from build123d import *

# Parameters (mm, degrees)
SKETCH1_R           = 100
SKETCH1_R_2         = 45
BOSS_EXTRUDE1_DEPTH = 60
SKETCH2_R           = 45
BOSS_EXTRUDE2_DEPTH = 15
CUT_EXTRUDE2_DEPTH  = 85
SKETCH5_R           = 70
CUT_EXTRUDE3_DEPTH  = 5
CUT_EXTRUDE4_DEPTH  = 50


with BuildPart() as part:
    # Sketch1 → Boss-Extrude1 (new body)
    with BuildSketch(Plane(origin=(0, 0, 0), x_dir=(1, 0, 0), z_dir=(0, 1, 0))):
        with Locations(Location((0, 0, 0), (0, 0, 270))):
            Circle(SKETCH1_R)
        with Locations(Location((0, 0, 0), (0, 0, 270))):
            Circle(SKETCH1_R_2, mode=Mode.SUBTRACT)
    extrude(amount=BOSS_EXTRUDE1_DEPTH)

    # Sketch2 → Boss-Extrude2 (add)
    with BuildSketch(Plane.XZ):
        with Locations(Location((0, 0, 0), (0, 0, 270))):
            Circle(SKETCH2_R)
    extrude(amount=-BOSS_EXTRUDE2_DEPTH)

    # Sketch4 → Cut-Extrude2 (cut)
    with BuildSketch(Plane(origin=(0, 60, 0), x_dir=(1, 0, 0), z_dir=(0, 1, 0))):
        with BuildLine():
            ThreePointArc((-4.583072667, 99.894922018), (-0.223462851, 98.100736099), (4.127927842, 99.914764733))
            ThreePointArc((4.127927842, 99.914764733), (-0.236423106, 103.790319504), (-4.583072667, 99.894922018))
        make_face()
        with BuildLine():
            ThreePointArc((29.85939598, 95.438024244), (33.342441429, 92.260966602), (38.051845487, 92.477332655))
            ThreePointArc((38.051845487, 92.477332655), (35.276214905, 97.611858812), (29.85939598, 95.438024244))
        make_face()
        with BuildLine():
            ThreePointArc((60.700380795, 79.469892232), (62.88675519, 75.293162907), (67.386148981, 73.885769439))
            ThreePointArc((67.386148981, 73.885769439), (66.534020776, 79.659967349), (60.700380795, 79.469892232))
        make_face()
        with BuildLine():
            ThreePointArc((84.220003843, 53.916518366), (84.845998166, 49.243892556), (88.592688393, 46.38249199))
            ThreePointArc((88.592688393, 46.38249199), (89.766841805, 52.099908168), (84.220003843, 53.916518366))
        make_face()
        with BuildLine():
            ThreePointArc((97.581451473, 21.860016662), (96.57156157, 17.255082), (99.113642097, 13.284801475))
            ThreePointArc((99.113642097, 13.284801475), (102.172456894, 18.255831149), (97.581451473, 21.860016662))
        make_face()
        with BuildLine():
            ThreePointArc((99.173135906, -12.833125672), (96.649169404, -16.814946103), (97.680027802, -21.415232161))
            ThreePointArc((97.680027802, -21.415232161), (102.254565777, -17.790168534), (99.173135906, -12.833125672))
        make_face()
        with BuildLine():
            ThreePointArc((88.80307651, -45.978403652), (85.069461017, -48.856843544), (84.464760551, -53.532272743))
            ThreePointArc((84.464760551, -53.532272743), (90.003264911, -51.690411336), (88.80307651, -45.978403652))
        make_face()
        with BuildLine():
            ThreePointArc((67.722055492, -73.578007583), (63.229120141, -75.005884603), (61.06179661, -79.19253118))
            ThreePointArc((61.06179661, -79.19253118), (66.896241989, -79.356027663), (67.722055492, -73.578007583))
        make_face()
        with BuildLine():
            ThreePointArc((38.472755112, -92.303017904), (33.762414213, -92.10810901), (30.293878822, -95.3010016))
            ThreePointArc((30.293878822, -95.3010016), (35.720545001, -97.450135883), (38.472755112, -92.303017904))
        make_face()
        with BuildLine():
            ThreePointArc((4.583072667, -99.894922018), (0.223462851, -98.100736099), (-4.127927842, -99.914764733))
            ThreePointArc((-4.127927842, -99.914764733), (0.236423106, -103.790319504), (4.583072667, -99.894922018))
        make_face()
        with BuildLine():
            ThreePointArc((-29.85939598, -95.438024244), (-33.342441429, -92.260966602), (-38.051845487, -92.477332655))
            ThreePointArc((-38.051845487, -92.477332655), (-35.276214905, -97.611858812), (-29.85939598, -95.438024244))
        make_face()
        with BuildLine():
            ThreePointArc((-60.700380795, -79.469892232), (-62.88675519, -75.293162907), (-67.386148981, -73.885769439))
            ThreePointArc((-67.386148981, -73.885769439), (-66.534020776, -79.659967349), (-60.700380795, -79.469892232))
        make_face()
        with BuildLine():
            ThreePointArc((-84.220003843, -53.916518366), (-84.845998166, -49.243892556), (-88.592688393, -46.38249199))
            ThreePointArc((-88.592688393, -46.38249199), (-89.766841805, -52.099908168), (-84.220003843, -53.916518366))
        make_face()
        with BuildLine():
            ThreePointArc((-97.581451473, -21.860016662), (-96.57156157, -17.255082), (-99.113642097, -13.284801475))
            ThreePointArc((-99.113642097, -13.284801475), (-102.172456894, -18.255831149), (-97.581451473, -21.860016662))
        make_face()
        with BuildLine():
            ThreePointArc((-99.173135906, 12.833125672), (-96.649169404, 16.814946103), (-97.680027802, 21.415232161))
            ThreePointArc((-97.680027802, 21.415232161), (-102.254565777, 17.790168534), (-99.173135906, 12.833125672))
        make_face()
        with BuildLine():
            ThreePointArc((-88.80307651, 45.978403652), (-85.069461017, 48.856843544), (-84.464760551, 53.532272743))
            ThreePointArc((-84.464760551, 53.532272743), (-90.003264911, 51.690411336), (-88.80307651, 45.978403652))
        make_face()
        with BuildLine():
            ThreePointArc((-67.722055492, 73.578007583), (-63.229120141, 75.005884603), (-61.06179661, 79.19253118))
            ThreePointArc((-61.06179661, 79.19253118), (-66.896241989, 79.356027663), (-67.722055492, 73.578007583))
        make_face()
        with BuildLine():
            ThreePointArc((-38.472755112, 92.303017904), (-33.762414213, 92.10810901), (-30.293878822, 95.3010016))
            ThreePointArc((-30.293878822, 95.3010016), (-35.720545001, 97.450135883), (-38.472755112, 92.303017904))
        make_face()
    extrude(amount=-CUT_EXTRUDE2_DEPTH, mode=Mode.SUBTRACT)

    # Sketch5 → Cut-Extrude3 (cut)
    with BuildSketch(Plane.XZ):
        with Locations(Location((0, 0, 0), (0, 0, 270))):
            Circle(SKETCH5_R)
    extrude(amount=-CUT_EXTRUDE3_DEPTH, mode=Mode.SUBTRACT)

    # Sketch3 → Cut-Extrude4 (cut)
    with BuildSketch(Plane(origin=(0, 15, 0), x_dir=(1, 0, 0), z_dir=(0, 1, 0))):
        with BuildLine():
            Line((-6.5, 1.5), (-5.291502622, 1.5))
            ThreePointArc((-5.291502622, 1.5), (5.5, 0), (-5.291502622, -1.5))
            Line((-5.291502622, -1.5), (-6.5, -1.5))
            Line((-6.5, -1.5), (-6.5, 1.5))
        make_face()
    extrude(amount=-CUT_EXTRUDE4_DEPTH, mode=Mode.SUBTRACT)


solid = part.part
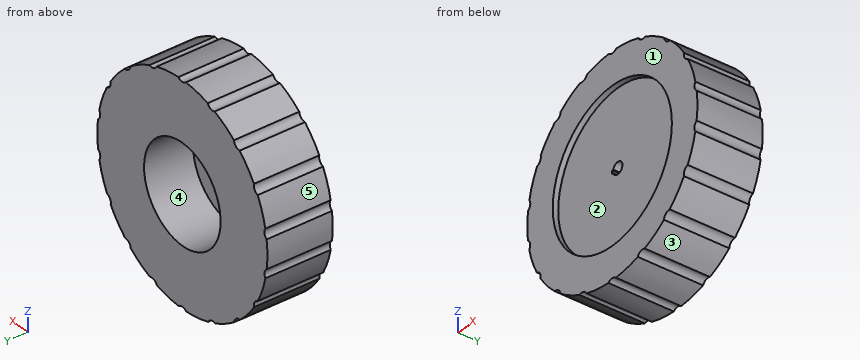
The model under review builds one solid part; all positions refer to its coordinate system, in mm. Face numbers are marked on the shaded views. A direction names the side the tool comes from. Coordinates: 2 decimals unless noted, no trailing zeros. Write each loop counter-clockwise with the first axis right and the second up, starting at its lowest first coordinate (ties: lowest second). Pieces come first, ordered by that corner, then holes. Notation, with made-up numbers: M 34,25 L 74,25 A27 cw 74,64 Z; hole C -6.5,27 d2. An arc over 180 degrees is marked long. Put each result on its own line as item: value.
1) Wall thickness on probe 1 along Z at (x, y) = (0, 10); probe 2 along X at (y, z) = (52, 0); probe 3 along X at (y, z) = (2, 0): over which ranges is each line inside the solid? List them lowest first. Write a range as [from, to].
Computed:
probe 1: z = [-98.11, -5.5], [5.5, 98.11]
probe 2: x = [-100, -45], [45, 100]
probe 3: x = [-100, -70], [70, 100]
2) Add section D-D on z = -26. Give the boundary of the cut face in (x, y).
Computed:
outline: M -96.56,0 L -64.99,0 L -64.99,5 L 64.99,5 L 64.99,0 L 96.56,0 L 96.56,60 L 36.73,60 L 36.73,15 L -36.73,15 L -36.73,60 L -96.56,60 Z
3) Add section B-B on z = -49. Give the boundary of the cut face in (x, y), then the cut area to 3 significant figures.
Computed:
outline: M -84.99,0 L -49.99,0 L -49.99,5 L 49.99,5 L 49.99,0 L 85,0 L 85,60 L -84.99,60 Z
area: 9,700 mm2
4) Add section C-C on x = 24. Give the boundary of the cut face in (y, z), then the cut area to 3 significant figures.
Computed:
outline: M 0,-97.08 L 60,-97.08 L 60,-38.07 L 15,-38.07 L 15,38.07 L 60,38.07 L 60,97.08 L 0,97.08 L 0,65.76 L 5,65.76 L 5,-65.76 L 0,-65.76 Z
area: 7,570 mm2
5) Add section A-A on x = 0. Give the boundary of the cut face in (y, z), then the cut area to 3 significant figures.
Computed:
outline: M 0,-98.11 L 60,-98.11 L 60,-45 L 15,-45 L 15,-5.5 L 5,-5.5 L 5,-70 L 0,-70 Z; M 0,70 L 5,70 L 5,5.5 L 15,5.5 L 15,45 L 60,45 L 60,98.11 L 0,98.11 Z
area: 6,910 mm2
6) For the marked faces 1 and 2, list the 3-axis set-ups (+Z, -Z, +X, -X, +Y, -Y) from which the entire face can be reached by the end or side of a thin tool; tool diameter is ignored.
Computed:
face 1: +Z, -Z, +X, -X, -Y
face 2: -Y
7) Clearance check with flat-ended pins moving along their axes: pin 1 Ø5 at (y, z) = (9.5, -11.5) entering from +X; pin 2 Ø14.5 at (x, z) = (0, 0) entering from -Y; pin 3 Ø10 at (x, y) = (66, 48) entering from +Z. State where each tip first meets the part, or that it passes through.
Computed:
pin 1: stops at x = 99.59
pin 2: stops at y = 5
pin 3: stops at z = 79.24
8) Draft analysis for pull direction Z (two halves, no side actions). For the marked faces 3, 4 and 5, state which applies: released by +Z, released by -Z, zero draft, split by the parting line, or undercut.
Computed:
face 3: released by -Z
face 4: undercut
face 5: released by +Z
